Geometry check sheet. Reference: drawing and pictorial views, mm from the part's lowest x, y, z. A direction names the side the tool comes from. Round coordinates to 2 decimals unless told otherwise and drop trailing zeros. Loops run counter-clockwise (first coordinate to the right, second up) from the corner with the lowest first, then second, coordinate; pieces in that order, holes last. Notation, with made-up numbers: (10, -17) -> (29, -17) arc R21 cw to (29, 17) -> close; hole circle Ø2 at (15.25, -13). An arc over 180 degrees is marked (long way). Use one line per item in the form item = value. Start each with the question number.
(1) Sectioned sample at C-C (x = 47.5). Record the cut outline in (y, z), and give its area (3 significant figures).
(2) Sectioned sample at A-A (x = 422.5). Record the cut outline in (y, z), and give its area (3 significant figures).
(3) Sectioned sample at B-B (y = 32). State how many separate pieces and enclosed holes the cut face has, and give its area (3 significant figures).
(4) Go/stop test with flat-tipped pins: pin 1 (6 mm diameter, centred on x = 78, z = 20.5, fed in from -Y); pin 2 (17.5 mm diameter, centred on x = 555, y = 32, fed in from -Z); pin 3 (17.5 mm diameter, centred on x = 25, y = 32, fed in from +Z); pin 4 (3 mm diameter, centred on x = 225.5, z = 6, fed in from +Y). Record where each tip stops, or that it passes through.
(5) Set-up check for the marked faces 1, 2 and 3: record each of +Z, -Z, +X, -X, +Y, -Y from which the full face is reachable in a straight line by a thin tool's end or side.
(6) Material ranges on probe 1 along Y at (x, z) = (290, 35); probe 2 along X at (y, z) = (215.5, 33.5); probe 3 along Z at (x, y) = (462, 15), recorded low to high. Write a range as [from, to].
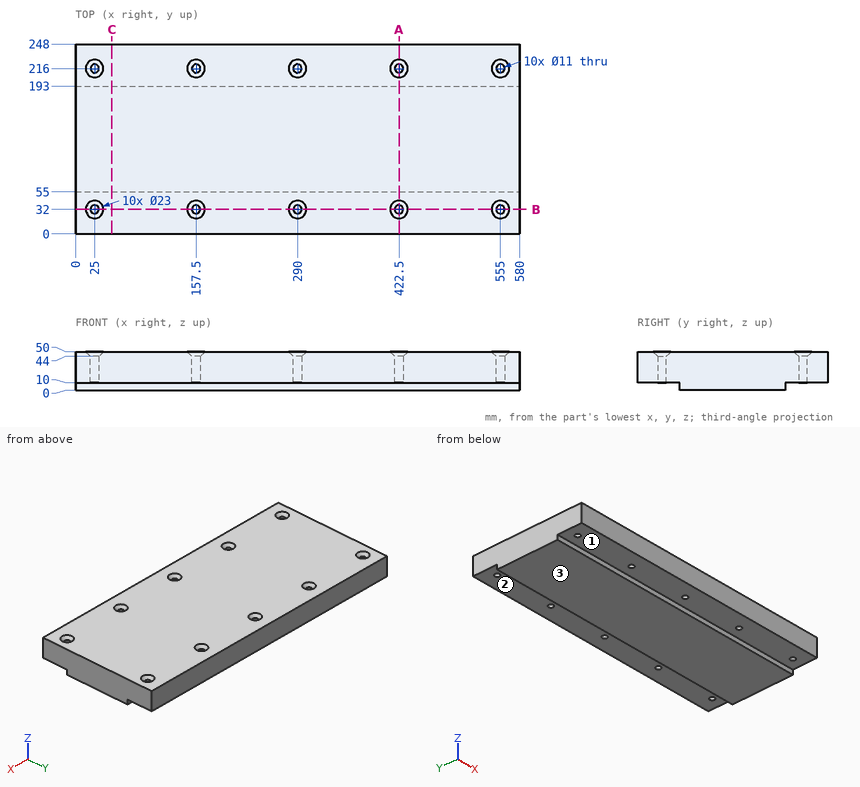
Checks:
q1.outline = (0, 10) -> (55, 10) -> (55, 0) -> (193, 0) -> (193, 10) -> (248, 10) -> (248, 50) -> (0, 50) -> close
q1.area = 11,300 mm2
q2.outline = (0, 10) -> (26.5, 10) -> (26.5, 44) -> (20.5, 50) -> (0, 50) -> close; (37.5, 10) -> (55, 10) -> (55, 0) -> (193, 0) -> (193, 10) -> (210.5, 10) -> (210.5, 44) -> (204.5, 50) -> (43.5, 50) -> (37.5, 44) -> close; (221.5, 10) -> (248, 10) -> (248, 50) -> (227.5, 50) -> (221.5, 44) -> close
q2.area = 10,300 mm2
q3.separate_pieces = 6
q3.enclosed_holes = 0
q3.area = 20,800 mm2
q4.pin_1 = 0
q4.pin_2 = 10
q4.pin_3 = 47.25
q4.pin_4 = 193
q5.face_1 = -Z, +X, -X, -Y
q5.face_2 = -Z, +X, -X, +Y
q5.face_3 = -Z, +X, -X, +Y, -Y
q6.probe_1 = [0, 26.5], [37.5, 210.5], [221.5, 248]
q6.probe_2 = [0, 19.52], [30.48, 152.02], [162.98, 284.52], [295.48, 417.02], [427.98, 549.52], [560.48, 580]
q6.probe_3 = [10, 50]
